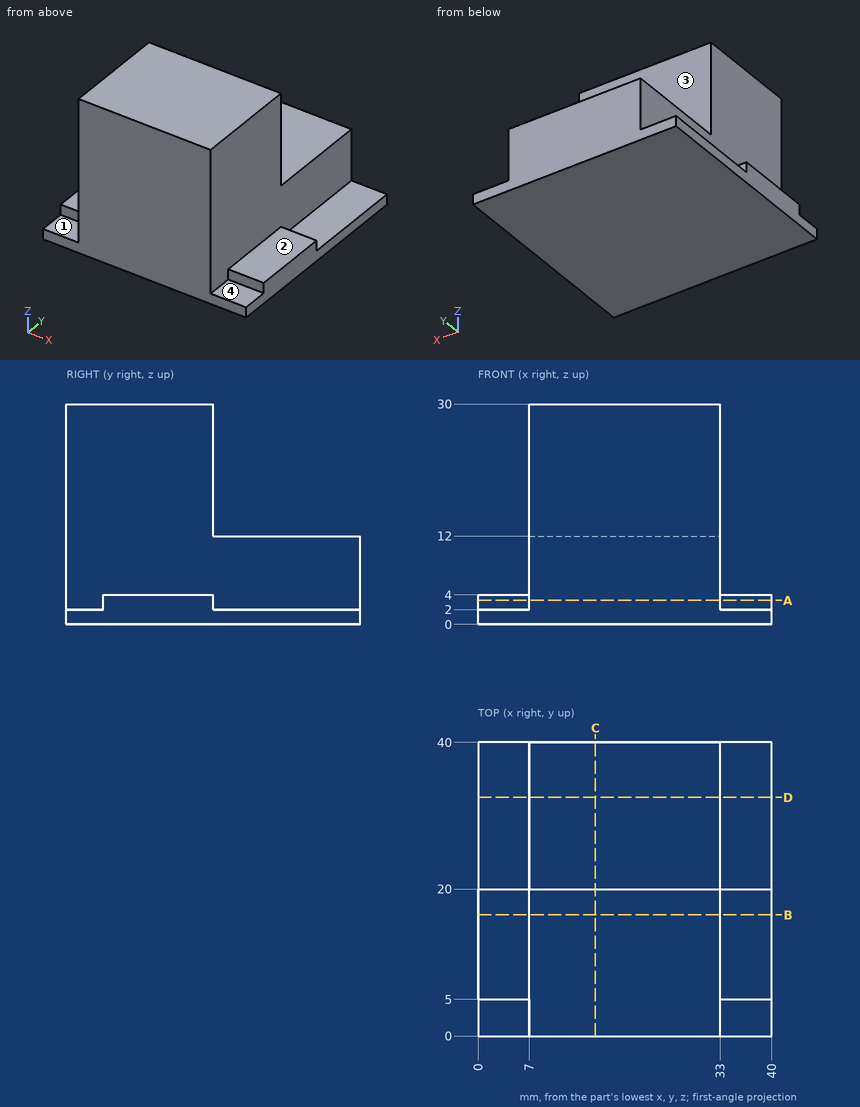
Here's the drawing with two shaded views (mm, measured from the low corner). I have some questions. A direction names the side the tool comes from. Coordinates: 2 decimals unless noted, no trailing zeros. Loops run counter-clockwise (first coordinate to the right, second up) from the corner with the lowest first, then second, coordinate; pieces in that order, holes last.
Item 1: Suppose I cut it at C-C (x = 16). Please give me the cut outline in (y, z).
Answers below:
outline: (0, 0) - (40, 0) - (40, 12) - (20, 12) - (20, 30) - (0, 30) - close
Item 2: Which directions (+Z, -Z, +X, -X, +Y, -Y) give clear straight access to the entire face, cutting with the end or side of a thin tool? Please do the marked faces 1, 2, 3 and 4.
Answers below:
face 1: +Z, -X, -Y
face 2: +Z, +X, +Y, -Y
face 3: +Z, +X, -X, +Y
face 4: +Z, +X, -Y
Item 3: Suppose I cut it at B-B (y = 16.5). Please give me the cut outline in (x, z).
Answers below:
outline: (0, 0) - (40, 0) - (40, 4) - (33, 4) - (33, 30) - (7, 30) - (7, 4) - (0, 4) - close
Item 4: Please list where these lines run through material, in increasing order: L1, parallel to X at y = 26.5, z = 8; L2, parallel to Z at x = 35, y = 32; L3, parallel to Y at x = 14, z = 17.
Answers below:
L1: x = 7 to 33
L2: z = 0 to 2
L3: y = 0 to 20
Item 5: I'm going to push flat-ended pins straight in: pin 1 (5.5 mm diameter, centred on x = 4, y = 15.5, fed in from +Z); pin 2 (1.6 mm diameter, centred on x = 2, z = 3, fed in from +Y); pin 3 (14 mm diameter, centred on y = 17, z = 15, fed in from -X). Where does each tip first touch, or does it pass through?
Answers below:
pin 1: stops at z = 4
pin 2: stops at y = 20
pin 3: stops at x = 7
Item 6: Suppose I cut it at A-A (z = 3.25). Please give me the cut outline in (x, y), then the cut area to 3 significant figures.
Answers below:
outline: (0, 5) - (7, 5) - (7, 0) - (33, 0) - (33, 5) - (40, 5) - (40, 20) - (33, 20) - (33, 40) - (7, 40) - (7, 20) - (0, 20) - close
area: 1,250 mm2
Item 7: Suppose I cut it at D-D (y = 32.5). Please give me the cut outline in (x, z).
Answers below:
outline: (0, 0) - (40, 0) - (40, 2) - (33, 2) - (33, 12) - (7, 12) - (7, 2) - (0, 2) - close
